Design review of the part shown in the three views and the two pictorial views. Dimensions are in mm from the part's minimum x, y and z. A direction names the side the tool comes from. Coordinates: 2 decimals unless noted, no trailing zeros. Order: outer loops, then holes, each group sorted by start corner. A loop starts at its lowest first (then second) coordinate and runs counter-clockwise, first axis right, second up. Notation, with made-up numbers: (13.25, 16.25) - (44.25, 16.25) arc R8 ccw to (44.25, 24.25) - close; hole circle Ø8 at (0, 13.25). An arc over 180 degrees is marked (long way). One line per item, written item: value. Start each with the question number.
(1) For the marked faces 4 and 5, list the 3-axis set-ups (+Z, -Z, +X, -X, +Y, -Y) from which the entire face can be reached by the end or side of a thin tool; tool diameter is ignored.
(2) Consider section C-C on z = 17.5. Write out the cut boundary in (x, y).
(3) Clearance check with flat-ended pins moving along their axes: pin 1 (4 mm diameter, centred on x = 35.5, y = 3.98, fed in from -Z); pin 2 (6 mm diameter, centred on y = 8, z = 9.5, fed in from +X). State where each tip first meets the part, or that it passes through.
(4) Consider section A-A on x = 35.5. Write out the cut boundary in (y, z), then the cut area to 3 significant figures.
(5) To check wall thickness, follow line 1 along Y through (x, z) = (35.5, 38); line 2 along Y through (x, z) = (2.95, 17.5); line 3 along X through (y, z) = (26, 38.6). State the ranges of each line that lie inside material, in increasing order.
(6) Mouldability with a two-part tool opening along Y and no side actions: class the marked faces 1, 2 and 3 as released by +Y, released by -Y, zero draft, split by the parting line, or undercut.
(7) Consider section D-D on y = 7.75. Write out the cut boundary in (x, z).
(8) Consider section B-B on y = 26. Write out the cut boundary in (x, z).
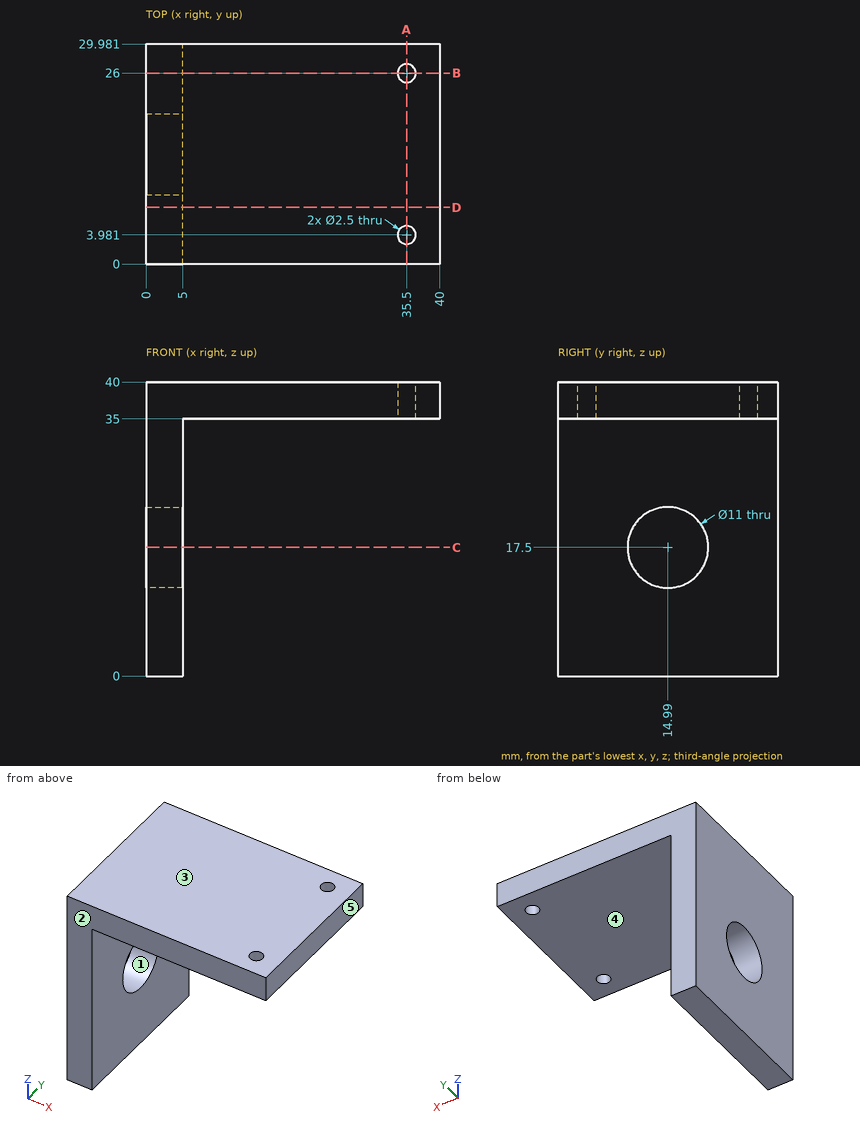
Geometry check:
1. face 4: -Z, +X, +Y, -Y
1. face 5: +Z, -Z, +X, +Y, -Y
2. outline: (0, 0) - (5, 0) - (5, 9.49) - (0, 9.49) - close; (0, 20.49) - (5, 20.49) - (5, 29.98) - (0, 29.98) - close
3. pin 1: stops at z = 35
3. pin 2: stops at x = 5
4. outline: (0, 35) - (2.73, 35) - (2.73, 40) - (0, 40) - close; (5.23, 35) - (24.75, 35) - (24.75, 40) - (5.23, 40) - close; (27.25, 35) - (29.98, 35) - (29.98, 40) - (27.25, 40) - close
4. area: 125 mm^2
5. line 1: y = 0 to 2.73, 5.23 to 24.75, 27.25 to 29.98
5. line 2: y = 0 to 9.49, 20.49 to 29.98
5. line 3: x = 0 to 34.25, 36.75 to 40
6. face 1: undercut
6. face 2: released by -Y
6. face 3: zero draft
7. outline: (0, 0) - (5, 0) - (5, 35) - (40, 35) - (40, 40) - (0, 40) - close
8. outline: (0, 0) - (5, 0) - (5, 35) - (34.25, 35) - (34.25, 40) - (0, 40) - close; (36.75, 35) - (40, 35) - (40, 40) - (36.75, 40) - close
